from build123d import *

# Parameters (mm, degrees)
BOSS_EXTRUDE1_DEPTH     = 1.6
CUT_EXTRUDE1_DEPTH      = 108.527298859
CUT_EXTRUDE1_DEPTH_BACK = 108.527298859
SKETCH2_OUTSIDE_W       = 52.356
SKETCH2_OUTSIDE_H       = 132.556
SKETCH2_OUTSIDE_W_2     = 49.825582729
SKETCH2_OUTSIDE_H_2     = 105


with BuildPart() as part:
    # Sketch1 → Boss-Extrude1 (new body)
    with BuildSketch(Plane(origin=(0, 0, 0), x_dir=(1, 0, 0), z_dir=(0, 1, 0))):
        Polygon((14, -1.6), (-14, -1.6), (-14, 1.6), (-9.75, 1.6), (-9.75, 5.9), (-14, 5.9), (-14, 9.1), (-9.75, 9.1), (-9.75, 13.4), (-14, 13.4), (-14, 16.6), (-9.75, 16.6), (-9.75, 20.9), (-14, 20.9), (-14, 24.1), (-9.75, 24.1), (-9.75, 28.4), (-14, 28.4), (-14, 31.6), (-9.75, 31.6), (-9.75, 35.9), (-14, 35.9), (-14, 39.1), (-9.75, 39.1), (-9.75, 43.4), (-14, 43.4), (-14, 46.6), (-9.75, 46.6), (-9.75, 50.9), (-14, 50.9), (-14, 54.1), (-9.75, 54.1), (-9.75, 58.4), (-14, 58.4), (-14, 61.6), (-9.75, 61.6), (-9.75, 65.9), (-14, 65.9), (-14, 69.1), (-9.75, 69.1), (-9.75, 73.4), (-14, 73.4), (-14, 76.6), (-9.75, 76.6), (-9.75, 80.9), (-14, 80.9), (-14, 84.1), (-9.75, 84.1), (-9.75, 88.4), (-14, 88.4), (-14, 91.6), (-9.75, 91.6), (-9.75, 95.9), (-14, 95.9), (-14, 99.1), (-9.75, 99.1), (-9.75, 103.4), (-14, 103.4), (-14, 106.6), (14, 106.6), (14, 103.4), (9.75, 103.4), (9.75, 99.1), (14, 99.1), (14, 95.9), (9.75, 95.9), (9.75, 91.6), (14, 91.6), (14, 88.4), (9.75, 88.4), (9.75, 84.1), (14, 84.1), (14, 80.9), (9.75, 80.9), (9.75, 76.6), (14, 76.6), (14, 73.4), (9.75, 73.4), (9.75, 69.1), (14, 69.1), (14, 65.9), (9.75, 65.9), (9.75, 61.6), (14, 61.6), (14, 58.4), (9.75, 58.4), (9.75, 54.1), (14, 54.1), (14, 50.9), (9.75, 50.9), (9.75, 46.6), (14, 46.6), (14, 43.4), (9.75, 43.4), (9.75, 39.1), (14, 39.1), (14, 35.9), (9.75, 35.9), (9.75, 31.6), (14, 31.6), (14, 28.4), (9.75, 28.4), (9.75, 24.1), (14, 24.1), (14, 20.9), (9.75, 20.9), (9.75, 16.6), (14, 16.6), (14, 13.4), (9.75, 13.4), (9.75, 9.1), (14, 9.1), (14, 5.9), (9.75, 5.9), (9.75, 1.6), (14, 1.6), align=None)
    extrude(amount=BOSS_EXTRUDE1_DEPTH)

    # Sketch2 outside → Cut-Extrude1 (cut, two sides: drawn at the far end of the back side and taken through both)
    with BuildSketch(Plane(origin=(0, 1.6, 0), x_dir=(1, 0, 0), z_dir=(0, 1, 0)).offset(-CUT_EXTRUDE1_DEPTH_BACK)):
        with Locations((0, 52.5)):
            Rectangle(SKETCH2_OUTSIDE_W, SKETCH2_OUTSIDE_H)
        with Locations((0.983399659, 52.5)):
            Rectangle(SKETCH2_OUTSIDE_W_2, SKETCH2_OUTSIDE_H_2, mode=Mode.SUBTRACT)
    extrude(amount=CUT_EXTRUDE1_DEPTH + CUT_EXTRUDE1_DEPTH_BACK, mode=Mode.SUBTRACT)


solid = part.part
CAD build for the part. Positions are in the model's coordinates, mm. Coordinates: 2 decimals unless noted, no trailing zeros. Write each loop counter-clockwise with the first axis right and the second up, starting at its lowest first coordinate (ties: lowest second). Pieces come first, ordered by that corner, then holes. Notation, with made-up numbers: (57, 82.5) - (74, 82.5) arc R17 cw to (74, 95.5) - close; hole circle Ø9 at (-38.5, 19.5). An arc over 180 degrees is marked (long way). Use a Markdown table: item, result. Add a question column.
Item 1: Drill centre line: L1, parallel to X at y = 1.2, z = -48.5. Where is it in solid material? Low to high. Write a range as from..to.
Item 2: Flat gauge pin, fed straight in: pin 1 (0.5 mm diameter, centred on y = 0.5, z = -71, fed in from +X). Where does the tip first touch, or does it go through?
Item 3: Band-saw the part on A-A, the plane x = -11.25. Give the number of separate pieces and of enclosed holes in the cut face, and give its area (3 significant figures).
Item 4: Band-saw the part on B-B, the plane z = -20. Give the cut face in (x, y), and give its area (3 significant figures).
Numbers:
| question | item | result |
|---|---|---|
| 1 | L1 | -9.75..9.75 |
| 2 | pin 1 | x = 9.75 |
| 3 | separate pieces | 15 |
| 3 | enclosed holes | 0 |
| 3 | area | 71.7 mm2 |
| 4 | outline | (-9.75, 0) - (9.75, 0) - (9.75, 1.6) - (-9.75, 1.6) - close |
| 4 | area | 31.2 mm2 |
